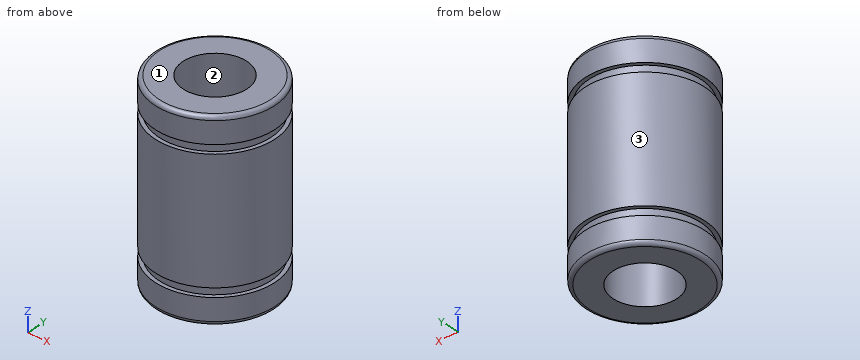
from build123d import *

# Parameters (mm, degrees)
F0_R     = 7.5
F0_R_2   = 4
F1_DEPTH = 24
F4_R     = 7.5
F4_R_2   = 7
F5_DEPTH = 1.1
F6_R     = 7.5
F6_R_2   = 7
F7_DEPTH = 1.1
F8_R     = 0.5


with BuildPart() as f1:
    # F0 (on Top) → F1 (new body)
    with BuildSketch(Plane.XY):
        Circle(F0_R)
        Circle(F0_R_2, mode=Mode.SUBTRACT)
    extrude(amount=F1_DEPTH)

    # F4 (on offset) → F5 (cut)
    with BuildSketch(Plane(origin=(0, 0, 3.25), x_dir=(1, 0, 0), z_dir=(0, 0, -1))):
        Circle(F4_R)
        Circle(F4_R_2, mode=Mode.SUBTRACT)
    extrude(amount=-F5_DEPTH, mode=Mode.SUBTRACT)

    # F6 (on offset) → F7 (cut)
    with BuildSketch(Plane.XY.offset(20.75)):
        Circle(F6_R)
        Circle(F6_R_2, mode=Mode.SUBTRACT)
    extrude(amount=-F7_DEPTH, mode=Mode.SUBTRACT)

    # F8
    f8_edges = [f1.edges().sort_by_distance(p)[0] for p in [
        (-7.5, 0, 24),
        (-7.5, 0, 0),
    ]]
    fillet(f8_edges, radius=F8_R)


solid = f1.part
The model under review builds one solid part; all positions refer to its coordinate system, in mm. Face numbers are marked on the shaded views. Give positions to 0.01 mm unless a question says otherwise; leave off trailing zeros. Order: outer loops, then holes, each group sorted by start corner. A loop starts at its lowest first (then second) coordinate and runs counter-clockwise, first axis right, second up. Notation, with made-up numbers: M -6.5,-2 L 35.5,-2 A23 ccw 35.5,7 Z; hole C 65.5,-4 d9. An arc over 180 degrees is marked long. Use one line per item in the form item = value. Start each with the question number.
Item 1: We need section C-C on z = 17.75. Give the boundary of the cut face in (x, y), plus the area to 3 significant figures.
Item 2: Insertion check: pin 1 Ø3 at (x, z) = (5.5, 3) entering from +Y; pin 2 Ø1 at (x, z) = (-3.5, 21) entering from -Y; pin 3 Ø3 at (y, z) = (3.5, 17) entering from -X. Each pin has a flat end and moves straight along its axis. Give the tip position at first contact, or say it passes through.
Item 3: We need section A-A on x = 0. Give the boundary of the cut face in (y, z).
Item 4: To check wall thickness, follow line 1 along Y through (x, z) = (0, 15.5); line 2 along X through (y, z) = (-2.5, 12.25); line 3 along Y through (x, z) = (-3.25, 16.5). State the ranges of each line that lie inside material, in increasing order. Write a range as from..to.
Item 5: The part is to be moulded in two halves that separate along X. For the marked faces 1, 2 and 3, say which applies: pulls with the +X half, pulls with the -X half, needs draft (parallel to the pull), parting line crosses it, or undercut.
Completed:
q1.outline = C 0,0 d15; hole C 0,0 d8
q1.area = 126 mm²
q2.pin_1 = 6.34
q2.pin_2 = -6.87
q2.pin_3 = -7.23
q3.outline = M -7.5,0.5 A0.5 ccw -7,0 L -4,0 L -4,24 L -7,24 A0.5 ccw -7.5,23.5 L -7.5,20.75 L -7,20.75 L -7,19.65 L -7.5,19.65 L -7.5,4.35 L -7,4.35 L -7,3.25 L -7.5,3.25 Z; M 4,0 L 7,0 A0.5 ccw 7.5,0.5 L 7.5,3.25 L 7,3.25 L 7,4.35 L 7.5,4.35 L 7.5,19.65 L 7,19.65 L 7,20.75 L 7.5,20.75 L 7.5,23.5 A0.5 ccw 7,24 L 4,24 Z
q4.line_1 = -7.5..-4, 4..7.5
q4.line_2 = -7.07..-3.12, 3.12..7.07
q4.line_3 = -6.76..-2.33, 2.33..6.76
q5.face_1 = needs draft
q5.face_2 = undercut
q5.face_3 = parting line crosses it
